```python
from build123d import *

# Parameters (mm, degrees)
BOSS_EXTRUDE1_DEPTH     = 5.75
CUT_EXTRUDE1_DEPTH      = 1
CUT_EXTRUDE1_DEPTH_BACK = 0.5
SKETCH2_W               = 12
SKETCH2_H               = 1.26
SKETCH2_W_2             = 10
FILLET1_R               = 0.1


with BuildPart() as part:
    # Sketch1 → Boss-Extrude1 (new, symmetric)
    with BuildSketch(Plane.XY):
        Polygon((5, 3.85), (5, 1.75), (14, 1.75), (14, 0), (5, 0), (0, 0), (0, 3.85), align=None)
    extrude(amount=BOSS_EXTRUDE1_DEPTH, both=True)

    # Sketch2 → Cut-Extrude1 (cut, two sides: drawn at the far end of the back side and taken through both)
    with BuildSketch(Plane(origin=(0, 1.75, 0), x_dir=(1, 0, 0), z_dir=(0, 1, 0)).offset(-CUT_EXTRUDE1_DEPTH_BACK)):
        with Locations((6, 3.78)):
            Rectangle(SKETCH2_W, SKETCH2_H)
        with Locations((5, 1.26)):
            Rectangle(SKETCH2_W_2, SKETCH2_H)
        with Locations((5, -1.26)):
            Rectangle(SKETCH2_W_2, SKETCH2_H)
        with Locations((6, -3.78)):
            Rectangle(SKETCH2_W, SKETCH2_H)
    extrude(amount=CUT_EXTRUDE1_DEPTH + CUT_EXTRUDE1_DEPTH_BACK, mode=Mode.SUBTRACT)

    # Fillet1
    fillet1_edges = [part.edges().sort_by_distance(p)[0] for p in [
        (0, 3.85, 0),
        (5, 3.85, 0),
        (14, 1.75, 0),
        (14, 0, 0),
        (0, 0, 0),
        (14, 0.875, 5.75),
        (9.5, 1.75, 5.75),
        (5, 2.8, 5.75),
        (2.5, 3.85, 5.75),
        (5, 2.75, 3.78),
        (5, 2.25, 3.15),
        (5, 2.25, 4.41),
        (5, 2.75, 1.26),
        (5, 2.25, 0.63),
        (5, 2.25, 1.89),
        (5, 2.75, -1.26),
        (5, 2.25, -1.89),
        (5, 2.25, -0.63),
        (5, 2.75, -3.78),
        (5, 2.25, -4.41),
        (5, 2.25, -3.15),
        (12, 1.75, 3.78),
        (10, 1.75, 1.26),
        (10, 1.75, -1.26),
        (12, 1.75, -3.78),
        (0, 1.925, 5.75),
        (0, 2, -3.15),
        (0, 2.75, -3.78),
        (0, 2, -4.41),
        (0, 1.25, -3.78),
        (8.5, 1.75, -3.15),
        (8.5, 1.75, -4.41),
        (0, 2, -0.63),
        (0, 2.75, -1.26),
        (0, 2, -1.89),
        (0, 1.25, -1.26),
        (7.5, 1.75, -0.63),
        (7.5, 1.75, -1.89),
        (0, 2, 1.89),
        (0, 2.75, 1.26),
        (7.5, 1.75, 1.89),
        (7.5, 1.75, 0.63),
        (0, 2, 0.63),
        (0, 1.25, 1.26),
        (2.5, 3.85, -5.75),
        (7, 0, 5.75),
        (0, 2, 4.41),
        (0, 2.75, 3.78),
        (8.5, 1.75, 4.41),
        (8.5, 1.75, 3.15),
        (0, 2, 3.15),
        (0, 1.25, 3.78),
        (5, 2.8, -5.75),
        (9.5, 1.75, -5.75),
        (14, 0.875, -5.75),
        (7, 0, -5.75),
        (0, 1.925, -5.75),
    ]]
    fillet(fillet1_edges, radius=FILLET1_R)


solid = part.part
```
The listing builds one solid part. Answer for the finished solid, in the listing's coordinates (mm). A direction names the side the tool comes from. Coordinates: 2 decimals unless noted, no trailing zeros. Loops run counter-clockwise (first coordinate to the right, second up) from the corner with the lowest first, then second, coordinate; pieces in that order, holes last. Notation, with made-up numbers: (-18.75, 23.25) -> (14.25, 23.25) arc R17 cw to (14.25, 48.25) -> close; hole circle Ø4 at (35, 52). An arc over 180 degrees is marked (long way). Use one line per item in the form item = value. Start each with the question number.
Item 1: A tool of negligible diameter and unlimited length cuts with its end or side. For faces 4 (the face through (2, 2.75, -1)), 5 (the face through (6, 1, -5.75)), 6 (the face through (3, 2, -1.89)), 7 (the face through (7, 0, 0)), 8 (the face through (5, 3, 0)), from which of +Z, -Z, +X, -X, +Y, -Y can it reach the whole face along a straight path? Write none if from no direction.
Item 2: The part is cut by section B-B on x = 1.5. Determine the outline of the cut face in (y, z).
Item 3: The mould has two halves that part along Z. Classify faces 1 (the face through (14, 1, 0)), 2 (the face through (2, 2.75, 4)), 3 (the face through (6, 1, 5.75)): released by +Z, released by -Z, zero draft, split by the parting line, or undercut.
Item 4: The part is cut by section A-A on z = -3.5. Determine the outline of the cut face in (x, y), then the cut area to 3 significant figures.
Item 5: Consider L1, parallel to Z at x = 4, y = 2.55; L2, parallel to Z at x = 10.5, y = 1.5; L3, parallel to Y at x = 4.5, z = 4. Determine where each line is inside the solid, lowest interval first. Write a range as [from, to].
Item 6: Flat-ended cylindrical pins translate along their axes: pin 1 Ø1.4 at (x, z) = (8, 4) entering from +Y; pin 2 Ø1 at (y, z) = (3, 2) entering from +X. Find the tip coordinate at first contact, or state that the pin passes through.
Answer key:
q1.face_4 = +X, -X
q1.face_5 = -Z, +X, -X, +Y, -Y
q1.face_6 = -X
q1.face_7 = +Z, -Z, +X, -X, -Y
q1.face_8 = +Z, -Z, +X, +Y
q2.outline = (0, -5.65) arc R0.1 ccw to (0.1, -5.75) -> (3.75, -5.75) arc R0.1 ccw to (3.85, -5.65) -> (3.85, 5.65) arc R0.1 ccw to (3.75, 5.75) -> (0.1, 5.75) arc R0.1 ccw to (0, 5.65) -> close; hole (1.25, -4.41) -> (2.75, -4.41) -> (2.75, -3.15) -> (1.25, -3.15) -> close; hole (1.25, -1.89) -> (2.75, -1.89) -> (2.75, -0.63) -> (1.25, -0.63) -> close; hole (1.25, 0.63) -> (2.75, 0.63) -> (2.75, 1.89) -> (1.25, 1.89) -> close; hole (1.25, 3.15) -> (2.75, 3.15) -> (2.75, 4.41) -> (1.25, 4.41) -> close
q3.face_1 = zero draft
q3.face_2 = undercut
q3.face_3 = released by +Z
q4.outline = (0, 0.1) arc R0.1 ccw to (0.1, 0) -> (13.9, 0) arc R0.1 ccw to (14, 0.1) -> (14, 1.65) arc R0.1 ccw to (13.9, 1.75) -> (12.1, 1.75) arc R0.1 ccw to (12, 1.65) -> (12, 1.25) -> (0.1, 1.25) arc R0.1 ccw to (0, 1.15) -> close; (0, 2.85) arc R0.1 ccw to (0.1, 2.75) -> (4.9, 2.75) arc R0.1 ccw to (5, 2.85) -> (5, 3.75) arc R0.1 ccw to (4.9, 3.85) -> (0.1, 3.85) arc R0.1 ccw to (0, 3.75) -> close
q4.area = 24.0 mm2
q5.L1 = [-5.75, -4.41], [-3.15, -1.89], [-0.63, 0.63], [1.89, 3.15], [4.41, 5.75]
q5.L2 = [-5.75, -4.41], [-3.15, 3.15], [4.41, 5.75]
q5.L3 = [0, 1.25], [2.75, 3.85]
q6.pin_1 = 1.75
q6.pin_2 = 5
